Input: part model. Units: mm. Frame: model coordinates. A direction names the side the tool comes from. Round coordinates to 2 decimals unless told otherwise and drop trailing zeros. Loops run counter-clockwise (first coordinate to the right, second up) from the corner with the lowest first, then second, coordinate; pieces in that order, holes last. Notation, with made-up numbers: (-37, 58.25) - (-29, 58.25) arc R21 cw to (-29, 87.25) - close; hole circle Ø11 at (7.5, 38). An arc over 180 degrees is marked (long way). One line per question, with ' | ' between items. Start each with the question number.
Item 1: Section C-C, the plane x = -7. Return loops of the section in (y, z).
Item 2: Section A-A, the plane z = -22.5. Return loops of the section in (x, y), plus the area to 3 significant figures.
Item 3: Material intervals for line 1 along Z through (x, y) = (1, -53); line 2 along Y through (x, z) = (-4.5, -22); line 3 along Z through (x, y) = (-10, -37.5), sorted ascending.
Item 4: Set-up query: faces 4 (the face through (-8.62, -17, 13)), 5 (the face through (11, -31, 20.874)), 6 (the face through (10, -61.156, -11)). Return all of +Z, -Z, +X, -X, +Y, -Y with unobstructed straight access to the full face (end or side cutting, diameter ignored); none if empty.
Item 5: First-contact query: pin 1 (5 mm diameter, centred on y = -14, z = -19, fed in from -X). Flat tip, straight axial feed; report the tip coordinate or a pass-through.
Item 6: Section B-B, the plane y = -48.5. Return loops of the section in (x, z), plus the area to 3 significant figures.
Item 7: Draft query along Y for faces 1 (the face through (10, -35, 8.174)), 2 (the face through (4, 0, -25)), 3 (the face through (29.48, -24, -35)). Return one class per face: pulls with the +Y half, pulls with the -Y half, needs draft (parallel to the pull), parting line crosses it, or undercut.
Item 8: Section D-D, the plane y = -7. Return loops of the section in (x, z), plus the area to 3 significant figures.
```python
from build123d import *

# Parameters (mm, degrees)
F1_DEPTH = 63.5
F2_W     = 50.8
F2_H     = 38.1
F3_DEPTH = 50.8


with BuildPart() as f1:
    # F0 (on Front) → F1 (new body)
    with BuildSketch(Plane.XZ):
        Polygon((-34.019788, -29.926063), (-34.019788, -55.326063), (29.480212, -55.326063), (29.480212, 20.873937), (-8.619788, 20.873937), (-8.619788, -29.926063), align=None)
    extrude(amount=F1_DEPTH)

    # F2 (on face) → F3 (cut)
    with BuildSketch(Plane(origin=(-8.619788, 0, 0), x_dir=(0, -1, 0), z_dir=(-1, 0, 0))):
        with Locations((35.755906, -10.876063)):
            Rectangle(F2_W, F2_H)
    extrude(amount=-F3_DEPTH, mode=Mode.SUBTRACT)


solid = f1.part
```
Return value:
1) outline: (-63.5, -55.33) - (0, -55.33) - (0, 20.87) - (-63.5, 20.87) - close; hole (-61.16, -29.93) - (-10.36, -29.93) - (-10.36, 8.17) - (-61.16, 8.17) - close
2) outline: (-8.62, -63.5) - (29.48, -63.5) - (29.48, -61.16) - (-8.62, -61.16) - close; (-8.62, -10.36) - (29.48, -10.36) - (29.48, 0) - (-8.62, 0) - close | area: 484 mm2
3) line 1: -55.33 to -29.93, 8.17 to 20.87 | line 2: -63.5 to -61.16, -10.36 to 0 | line 3: -55.33 to -29.93
4) face 4: +Z, -X, +Y, -Y | face 5: +Z, +X, -X, +Y, -Y | face 6: +X, -X
5) pin 1: through
6) outline: (-34.02, -55.33) - (29.48, -55.33) - (29.48, -29.93) - (-34.02, -29.93) - close; (-8.62, 8.17) - (29.48, 8.17) - (29.48, 20.87) - (-8.62, 20.87) - close | area: 2,100 mm2
7) face 1: undercut | face 2: pulls with the +Y half | face 3: needs draft
8) outline: (-34.02, -55.33) - (29.48, -55.33) - (29.48, 20.87) - (-8.62, 20.87) - (-8.62, -29.93) - (-34.02, -29.93) - close | area: 3,550 mm2
